from build123d import *

# Parameters (mm, degrees)
SKETCH1_W               = 70
SKETCH1_H               = 82
BOSS_EXTRUDE1_DEPTH     = 4.5
SKETCH2_W               = 4.5
SKETCH2_H               = 70
BOSS_EXTRUDE2_DEPTH     = 120
BOSS_EXTRUDE3_DEPTH     = 20
CUT_EXTRUDE1_REACH      = 137.67
SKETCH4_R               = 27.5
CUT_EXTRUDE2_REACH      = 152.77
SKETCH5_R               = 3.5
SKETCH6_W               = 6
SKETCH6_H               = 8
BOSS_EXTRUDE4_DEPTH     = 3
SKETCH7_W               = 6
SKETCH7_H               = 8
BOSS_EXTRUDE5_DEPTH     = 3
CUT_EXTRUDE4_DEPTH      = 116.905133622
CUT_EXTRUDE4_DEPTH_BACK = 116.905133622
SKETCH8_R               = 1.55
FILLET1_R               = 2.5
SKETCH9_W               = 30.5
SKETCH9_H               = 40.5
BOSS_EXTRUDE6_DEPTH     = 9


with BuildPart() as part:
    # Sketch1 → Boss-Extrude1 (new body)
    with BuildSketch(Plane(origin=(0, 0, 0), x_dir=(0, 1, 0), z_dir=(0, 0, 1))):
        Rectangle(SKETCH1_W, SKETCH1_H)
    extrude(amount=BOSS_EXTRUDE1_DEPTH)

    # Sketch2 → Boss-Extrude2 (add)
    with BuildSketch(Plane.XY.offset(4.5)):
        with Locations((38.75, 0)):
            Rectangle(SKETCH2_W, SKETCH2_H)
    extrude(amount=BOSS_EXTRUDE2_DEPTH)

    # Sketch3 → Boss-Extrude3 (add)
    with BuildSketch(Plane.XY.offset(4.5)):
        Polygon((36.5, 35), (-41, 35), (-41, -35), (36.5, -35), (36.5, -30.5), (-36.5, -30.5), (-36.5, 30.5), (36.5, 30.5), align=None)
    extrude(amount=BOSS_EXTRUDE3_DEPTH)

    # Sketch4 → Cut-Extrude1 (cut, up to next)
    with BuildSketch(Plane(origin=(0, 0, 0), x_dir=(1, 0, 0), z_dir=(0, 0, -1)), mode=Mode.PRIVATE) as cut_extrude1_sk1:
        with Locations(Location((0, 0, 0), (0, 0, 180))):
            Circle(SKETCH4_R)
    cut_extrude1_tool1 = extrude(cut_extrude1_sk1.sketch, amount=-CUT_EXTRUDE1_REACH, mode=Mode.PRIVATE) & part.part
    add(cut_extrude1_tool1.solids().sort_by_distance((0, 0, 0))[0], mode=Mode.SUBTRACT)

    # Sketch5 → Cut-Extrude2 (cut, up to next)
    with BuildSketch(Plane(origin=(36.5, 0, 0), x_dir=(0, -1, 0), z_dir=(-1, 0, 0)), mode=Mode.PRIVATE) as cut_extrude2_sk1:
        with Locations((0, 38)):
            Circle(SKETCH5_R)
    cut_extrude2_tool1 = extrude(cut_extrude2_sk1.sketch, amount=-CUT_EXTRUDE2_REACH, mode=Mode.PRIVATE) & part.part
    # Sketch5 → Cut-Extrude2 (cut, up to next)
    with BuildSketch(Plane(origin=(36.5, 0, 0), x_dir=(0, -1, 0), z_dir=(-1, 0, 0)), mode=Mode.PRIVATE) as cut_extrude2_sk2:
        with BuildLine():
            Line((-7.5, 124.5), (7.5, 124.5))
            Line((7.5, 124.5), (7.5, 109.5))
            ThreePointArc((7.5, 109.5), (0, 102), (-7.5, 109.5))
            Line((-7.5, 109.5), (-7.5, 124.5))
        make_face()
    cut_extrude2_tool2 = extrude(cut_extrude2_sk2.sketch, amount=-CUT_EXTRUDE2_REACH, mode=Mode.PRIVATE) & part.part
    add(cut_extrude2_tool1.solids().sort_by_distance((36.5, 0, 38))[0], mode=Mode.SUBTRACT)
    add(cut_extrude2_tool2.solids().sort_by_distance((36.5, 0, 113.987689))[0], mode=Mode.SUBTRACT)

    # Sketch6 → Boss-Extrude4 (add)
    with BuildSketch(Plane.XY.offset(124.5)):
        with Locations((44, 29)):
            Rectangle(SKETCH6_W, SKETCH6_H)
        with Locations((44, -29)):
            Rectangle(SKETCH6_W, SKETCH6_H)
    extrude(amount=-BOSS_EXTRUDE4_DEPTH)

    # Sketch7 → Boss-Extrude5 (add)
    with BuildSketch(Plane.XY.offset(24.5)):
        with Locations((-44, -29)):
            Rectangle(SKETCH7_W, SKETCH7_H)
        with Locations((-44, 29)):
            Rectangle(SKETCH7_W, SKETCH7_H)
    extrude(amount=-BOSS_EXTRUDE5_DEPTH)

    # Sketch8 → Cut-Extrude4 (cut, two sides: drawn at the far end of the back side and taken through both)
    with BuildSketch(Plane.XY.offset(24.5).offset(-CUT_EXTRUDE4_DEPTH_BACK)):
        with Locations((-44, 29)):
            Circle(SKETCH8_R)
        with Locations((44, 29)):
            Circle(SKETCH8_R)
        with Locations((44, -29)):
            Circle(SKETCH8_R)
        with Locations((-44, -29)):
            Circle(SKETCH8_R)
    extrude(amount=CUT_EXTRUDE4_DEPTH + CUT_EXTRUDE4_DEPTH_BACK, mode=Mode.SUBTRACT)

    # Fillet1
    # the kernel refuses this fillet: 2.5 mm, written as the material it adds along each edge
    with BuildSketch(Plane(origin=(-41, 33, 24.5), x_dir=(-1.5774048733869181e-12, 1.0, 0), z_dir=(0, 0, -1)), Plane(origin=(41, -33, 124.5), x_dir=(1.5312195955625318e-12, -1.0, 0), z_dir=(0, 0, -1))) as fillet1_piece_1:
        with BuildLine():
            CenterArc((2.5, -2.449489743), FILLET1_R, 101.536959033, 78.463040967)
            Line((0, -2.449489743), (0, 0))
            Line((0, 0), (2, 0))
        make_face()
    extrude(amount=3)
    with BuildSketch(Plane(origin=(-41, 25, 24.5), x_dir=(0, -1, 0), z_dir=(0, 0, -1)), Plane(origin=(41, -25, 124.5), x_dir=(0, 1, 0), z_dir=(0, 0, -1))) as fillet1_piece_2:
        with BuildLine():
            CenterArc((FILLET1_R, FILLET1_R), FILLET1_R, 180, 90)
            Line((0, FILLET1_R), (0, 0))
            Line((0, 0), (FILLET1_R, 0))
        make_face()
    extrude(amount=3)
    with BuildSketch(Plane(origin=(-41, -25, 24.5), x_dir=(0, 1, 0), z_dir=(0, 0, -1)), Plane(origin=(41, 25, 124.5), x_dir=(0, -1, 0), z_dir=(0, 0, -1))) as fillet1_piece_3:
        with BuildLine():
            CenterArc((FILLET1_R, -FILLET1_R), FILLET1_R, 90, 90)
            Line((0, -FILLET1_R), (0, 0))
            Line((0, 0), (FILLET1_R, 0))
        make_face()
    extrude(amount=3)
    with BuildSketch(Plane(origin=(-41, -33, 24.5), x_dir=(-1.6022738691384966e-12, -1.0, 0), z_dir=(0, 0, -1)), Plane(origin=(41, 33, 124.5), x_dir=(1.4885870314169656e-12, 1.0, 0), z_dir=(0, 0, -1))) as fillet1_piece_4:
        with BuildLine():
            CenterArc((2.5, 2.449489743), FILLET1_R, 180, 78.463040967)
            Line((0, 2.449489743), (0, 0))
            Line((0, 0), (2, 0))
        make_face()
    extrude(amount=3)
    # the kernel refuses this fillet: 2.5 mm, written as the material it takes off along each edge
    with BuildSketch(Plane(origin=(-47, 25, 30.75), x_dir=(1, 0, 0), z_dir=(0, 0, -1)), Plane(origin=(-47, 33, 30.75), x_dir=(0, -1, 0), z_dir=(0, 0, -1)), Plane(origin=(-47, -33, 30.75), x_dir=(1, 0, 0), z_dir=(0, 0, -1)), Plane(origin=(-47, -25, 30.75), x_dir=(0, -1, 0), z_dir=(0, 0, -1)), Plane(origin=(47, 33, 130.75), x_dir=(-1, 0, 0), z_dir=(0, 0, -1)), Plane(origin=(47, 25, 130.75), x_dir=(0, 1, 0), z_dir=(0, 0, -1))) as fillet1_2_piece_1:
        with BuildLine():
            CenterArc((FILLET1_R, -FILLET1_R), FILLET1_R, 90, 90)
            Line((0, -FILLET1_R), (0, 0))
            Line((0, 0), (FILLET1_R, 0))
        make_face()
    extrude(amount=15.5, mode=Mode.SUBTRACT)
    with BuildSketch(Plane(origin=(47, -25, 130.75), x_dir=(0, -1, 0), z_dir=(0, 0, -1)), Plane(origin=(47, -33, 130.75), x_dir=(-1, 0, 0), z_dir=(0, 0, -1))) as fillet1_2_piece_2:
        with BuildLine():
            CenterArc((FILLET1_R, FILLET1_R), FILLET1_R, 180, 90)
            Line((0, FILLET1_R), (0, 0))
            Line((0, 0), (FILLET1_R, 0))
        make_face()
    extrude(amount=15.5, mode=Mode.SUBTRACT)

    # Sketch9 → Boss-Extrude6 (add)
    with BuildSketch(Plane(origin=(36.5, 0, 0), x_dir=(0, -1, 0), z_dir=(-1, 0, 0))):
        Polygon((-30.5, 24.5), (-30.5, 68), (30.5, 68), (30.5, 24.5), (30.5, 4.5), (-30.5, 4.5), align=None)
        with Locations((0, 38)):
            Rectangle(SKETCH9_W, SKETCH9_H, mode=Mode.SUBTRACT)
    extrude(amount=BOSS_EXTRUDE6_DEPTH)


solid = part.part
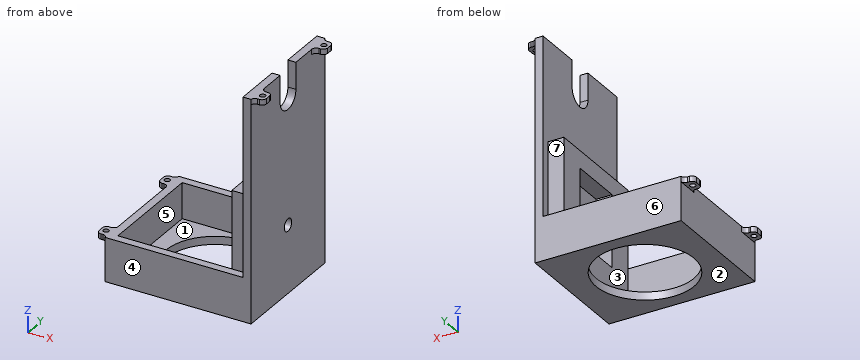
The listing builds one solid part. Answer for the finished solid, in the listing's coordinates (mm). Face numbers are marked on the shaded views. A direction names the side the tool comes from. Coordinates: 2 decimals unless noted, no trailing zeros. Loops run counter-clockwise (first coordinate to the right, second up) from the corner with the lowest first, then second, coordinate; pieces in that order, holes last.
1) Flat-ended cylindrical pins translate along their axes: pin 1 Ø10 at (x, y) = (-25, 18.5) entering from +Z; pin 2 Ø4 at (x, y) = (-44, -29) entering from -Z; pin 3 Ø10 at (x, z) = (31, 39) entering from -Y. Find the tip coordinate at first contact, or state that the pin passes through.
2) Find section B-B on z = 38. Write down the section's boundary in (x, y), then the cut area to 3 significant figures.
3) Find section D-D on x = -29. Write down the section's boundary in (y, z), then the cut area to 3 significant figures.
4) Determine the mould class of the marked faces 1, 2, 3 and 4 for opening direction Y: pulls with the +Y half, pulls with the -Y half, needs draft (parallel to the pull), parting line crosses it, or undercut.
5) Find section A-A on y = -29. Write down the section's boundary in (x, z).
6) Find the intervals of material crossed by L1, parallel to Y at x = -44, z = 22; L2, parallel to X at y = -29, z = 23.45; L3, parallel to Y at x = -31, z = 12.5, in increasing order.
7) A tool of negligible diameter and unlimited length cuts with its end or side. For the marked faces 5, 6 and 7, from which of +Z, -Z, +X, -X, +Y, -Y can it reach the whole face along a straight path? Write none if from no direction.
8) Find section C-C on x = -11. Write down the section's boundary in (y, z), then the cut area to 3 significant figures.
Values:
1. pin 1: stops at z = 4.5
1. pin 2: stops at z = 21.5
1. pin 3: stops at y = -30.5
2. outline: (27.5, -30.5) - (36.5, -30.5) - (36.5, -35) - (41, -35) - (41, -3.5) - (36.5, -3.5) - (36.5, -15.25) - (27.5, -15.25) - close; (27.5, 15.25) - (36.5, 15.25) - (36.5, 3.5) - (41, 3.5) - (41, 35) - (36.5, 35) - (36.5, 30.5) - (27.5, 30.5) - close
2. area: 558 mm2
3. outline: (-35, 0) - (35, 0) - (35, 24.5) - (30.5, 24.5) - (30.5, 4.5) - (-30.5, 4.5) - (-30.5, 24.5) - (-35, 24.5) - close
3. area: 495 mm2
4. face 1: undercut
4. face 2: needs draft
4. face 3: undercut
4. face 4: pulls with the -Y half
5. outline: (-47, 21.5) - (-45.55, 21.5) - (-45.55, 24.5) - (-47, 24.5) - close; (-42.45, 21.5) - (-41, 21.5) - (-41, 0) - (41, 0) - (41, 121.5) - (42.45, 121.5) - (42.45, 124.5) - (36.5, 124.5) - (36.5, 68) - (27.5, 68) - (27.5, 4.5) - (-36.5, 4.5) - (-36.5, 24.5) - (-42.45, 24.5) - close; (45.55, 121.5) - (47, 121.5) - (47, 124.5) - (45.55, 124.5) - close
6. L1: y = -33 to -30.55, -27.45 to -25, 25 to 27.45, 30.55 to 33
6. L2: x = -47 to -45.55, -42.45 to -36.5, 27.5 to 41
6. L3: y = -35 to -30.5, 30.5 to 35
7. face 5: +Z
7. face 6: +Z, -Z, +X, -X, +Y
7. face 7: +Z, -X, +Y
8. outline: (-35, 0) - (-25.2, 0) - (-25.2, 4.5) - (-30.5, 4.5) - (-30.5, 24.5) - (-35, 24.5) - close; (25.2, 0) - (35, 0) - (35, 24.5) - (30.5, 24.5) - (30.5, 4.5) - (25.2, 4.5) - close
8. area: 268 mm2
